```python
from build123d import *

# Parameters (mm, degrees)
CROQUIS1_R              = 3
SALIENTE_EXTRUIR1_DEPTH = 4


with BuildPart() as part:
    # Croquis1 → Saliente-Extruir1 (new body)
    with BuildSketch(Plane.XY):
        Polygon((5.2, 3), (5.2, 9), (0, 12), (-5.2, 9), (-5.2, 3), (0, 0), align=None)
        with Locations((0, 6)):
            Circle(CROQUIS1_R, mode=Mode.SUBTRACT)
    extrude(amount=SALIENTE_EXTRUIR1_DEPTH)


solid = part.part
```
The model under review builds one solid part; all positions refer to its coordinate system, in mm. Round coordinates to 2 decimals unless told otherwise and drop trailing zeros. Write each loop counter-clockwise with the first axis right and the second up, starting at its lowest first coordinate (ties: lowest second). Pieces come first, ordered by that corner, then holes. Notation, with made-up numbers: (76, -16) - (81, -16) arc R16 cw to (81, -10) - close; hole circle Ø3 at (-13.5, -36.75). An arc over 180 degrees is marked (long way). Answer as CSV lines item,"result". Start each with the question number.
(1) To check wall thickness, follow line 1 (Y direction, x = -1.5, z = 2.45); line 2 (X direction, y = 8.25, z = 1.2); line 3 (X direction, y = 8.5, z = 1.6). State the ranges of each line that lie inside material, in increasing order.
(2) Draft analysis for pull direction Y (two halves, no side actions). For faces 1 (the flat face through (-2.6, 10.5, 2)), 2 (the flat face through (2.6, 1.5, 2)), 3 (the cylindrical face through (-0.65, 3.07, 1.97)), 4 (the flat face through (-5.2, 6, 2)), state which applies: pulls with the +Y half, pulls with the -Y half, needs draft (parallel to the pull), parting line crosses it, or undercut.
(3) For pin 1 Ø1.5 at (x, y) = (-3, 10.5) entering from +Z, flat-tipped, find the tip position at first contact; note if it passes through.
(4) We need section A-A on y = 6. State the section outline as (x, z) points.
(5) We need section D-D on y = 9.25. State the section outline as (x, z) points, plus the area to 3 significant figures.
(6) We need section C-C on x = -2.5. State the section outline as (y, z) points.
(7) We need section B-B on z = 1.55. State the section outline as (x, y) points, plus the area to 3 significant figures.
Worked answers:
1,line 1,"0.87 to 3.4, 8.6 to 11.13"
1,line 2,"-5.2 to -1.98, 1.98 to 5.2"
1,line 3,"-5.2 to -1.66, 1.66 to 5.2"
2,face 1,"pulls with the +Y half"
2,face 2,"pulls with the -Y half"
2,face 3,"undercut"
2,face 4,"needs draft"
3,pin 1,"z = 4"
4,outline,"(-5.2, 0) - (-3, 0) - (-3, 4) - (-5.2, 4) - close; (3, 0) - (5.2, 0) - (5.2, 4) - (3, 4) - close"
5,outline,"(-4.77, 0) - (4.77, 0) - (4.77, 4) - (-4.77, 4) - close"
5,area,"38.1 mm²"
6,outline,"(1.44, 0) - (4.34, 0) - (4.34, 4) - (1.44, 4) - close; (7.66, 0) - (10.56, 0) - (10.56, 4) - (7.66, 4) - close"
7,outline,"(-5.2, 3) - (0, 0) - (5.2, 3) - (5.2, 9) - (0, 12) - (-5.2, 9) - close; hole circle Ø6 at (0, 6)"
7,area,"65.3 mm²"
